```python
from build123d import *

# Parameters (mm, degrees)
SKETCH_1_W                                 = 300
SKETCH_1_H                                 = 120
EXTRUDE_1_DEPTH                            = 100
EXTRUDE_2_DEPTH                            = 20
FILLET_2_R                                 = 10
FILLET_3_R                                 = 10
MIRROR_6_AT_THE_SECOND_PLANE_COPY_1_DEPTH  = 20
FILLET_10_R                                = 10
FILLET_11_R                                = 10
FILLET_12_R                                = 10
FILLET_13_R                                = 10
FILLET_14_R                                = 10
FILLET_15_R                                = 10
CUT_EXTRUDE_1_REACH                        = 258.744
PATTERN_LINEAR_1_COUNT                     = 4
PATTERN_LINEAR_1_PITCH                     = 40
PATTERN_LINEAR_1_COL_COUNT                 = 4
PATTERN_LINEAR_1_COL_PITCH                 = 40
SKETCH_4_R                                 = 30
EXTRUDE_3_DEPTH                            = 13
SKETCH_6_R                                 = 32.5
CUT_EXTRUDE_2_DEPTH                        = 283.853914089
FILLET_16_R                                = 5
CUT_EXTRUDE_6_DEPTH                        = 399.453619326
CUT_EXTRUDE_6_DEPTH_BACK                   = 10
SKETCH_10_W                                = 239.935229407
SKETCH_10_H                                = 310.477115034
SKETCH_11_R                                = 2
CUT_EXTRUDE_7_DEPTH                        = 10
MIRROR_8_AT_THE_SECOND_PLANE_COPY_1_SKET_R = 2
MIRROR_8_AT_THE_SECOND_PLANE_COPY_1_DEPTH  = 10
SKETCH_12_R                                = 2
CUT_EXTRUDE_8_DEPTH                        = 261.089093804
PATTERN_CIRCULAR_2_COUNT                   = 6


with BuildPart() as part:
    # 草图1 → 凸台-拉伸1 (new body)
    with BuildSketch(Plane.XY):
        Rectangle(SKETCH_1_W, SKETCH_1_H)
    extrude(amount=EXTRUDE_1_DEPTH)

    # 草图2 → 凸台-拉伸2 (add)
    with BuildSketch(Plane(origin=(0, 60, 0), x_dir=(1, 0, 0), z_dir=(0, 1, 0))):
        with BuildLine():
            Line((150, -50), (150, -40))
            ThreePointArc((150, -40), (228.729833462, -50), (150, -60))
            Line((150, -60), (150, -50))
        make_face()
    extrude_2 = extrude(amount=-EXTRUDE_2_DEPTH)

    # 圆角2
    fillet_2_edges = [part.edges().sort_by_distance(p)[0] for p in [
        (150, 50, 40),
    ]]
    fillet(fillet_2_edges, radius=FILLET_2_R)

    # 圆角3
    fillet_3_edges = [part.edges().sort_by_distance(p)[0] for p in [
        (150, 50, 60),
    ]]
    fillet(fillet_3_edges, radius=FILLET_3_R)

    # 镜向6: 凸台-拉伸2 across plane
    add(extrude_2.mirror(Plane(origin=(0, 0, 0), x_dir=(0, 0, 1), z_dir=(1, 0, 0))))

    # 镜向6 at the second plane: 凸台-拉伸2 across plane
    add(extrude_2.mirror(Plane.ZX))

    # 镜向6 at the second plane copy 1 sket → 镜向6 at the second plane copy 1 (add)
    with BuildSketch(Plane(origin=(0, -60, 0), x_dir=(-1, 0, 0), z_dir=(0, -1, 0))):
        with BuildLine():
            Line((150, -50), (150, -40))
            ThreePointArc((150, -40), (228.729833462, -50), (150, -60))
            Line((150, -60), (150, -50))
        make_face()
    extrude(amount=-MIRROR_6_AT_THE_SECOND_PLANE_COPY_1_DEPTH)

    # 圆角10
    fillet_10_edges = [part.edges().sort_by_distance(p)[0] for p in [
        (150, -50, 60),
    ]]
    fillet(fillet_10_edges, radius=FILLET_10_R)

    # 圆角11
    fillet_11_edges = [part.edges().sort_by_distance(p)[0] for p in [
        (150, -50, 40),
    ]]
    fillet(fillet_11_edges, radius=FILLET_11_R)

    # 圆角12
    fillet_12_edges = [part.edges().sort_by_distance(p)[0] for p in [
        (-150, 50, 40),
    ]]
    fillet(fillet_12_edges, radius=FILLET_12_R)

    # 圆角13
    fillet_13_edges = [part.edges().sort_by_distance(p)[0] for p in [
        (-150, -50, 60),
    ]]
    fillet(fillet_13_edges, radius=FILLET_13_R)

    # 圆角14
    fillet_14_edges = [part.edges().sort_by_distance(p)[0] for p in [
        (-150, 50, 60),
    ]]
    fillet(fillet_14_edges, radius=FILLET_14_R)

    # 圆角15
    fillet_15_edges = [part.edges().sort_by_distance(p)[0] for p in [
        (-150, -50, 40),
    ]]
    fillet(fillet_15_edges, radius=FILLET_15_R)

    # 草图3 → 切除-拉伸1 (cut, up to next)
    with BuildSketch(Plane.XY.offset(100), mode=Mode.PRIVATE) as cut_extrude_1_sk1:
        with BuildLine():
            Line((-11.916195323, -32.511613), (-11.916195323, 32.511613))
            ThreePointArc((-11.916195323, 32.511613), (0, 44.427808323), (11.916195323, 32.511613))
            Line((11.916195323, 32.511613), (11.916195323, -32.511613))
            ThreePointArc((11.916195323, -32.511613), (0, -44.427808323), (-11.916195323, -32.511613))
        make_face()
    cut_extrude_1_tool1 = extrude(cut_extrude_1_sk1.sketch, amount=-CUT_EXTRUDE_1_REACH, mode=Mode.PRIVATE) & part.part
    cut_extrude_1 = cut_extrude_1_tool1.solids().sort_by_distance((0, 0, 100))[0]
    add(cut_extrude_1, mode=Mode.SUBTRACT)

    # 阵列(线性)1: 切除-拉伸1 ×4
    with Locations(*[(i * PATTERN_LINEAR_1_PITCH, 0, 0) for i in range(1, PATTERN_LINEAR_1_COUNT)]):
        add(cut_extrude_1, mode=Mode.SUBTRACT)

    # 阵列(线性)1 col: 切除-拉伸1 ×4
    with Locations(*[(-i * PATTERN_LINEAR_1_COL_PITCH, 0, 0) for i in range(1, PATTERN_LINEAR_1_COL_COUNT)]):
        add(cut_extrude_1, mode=Mode.SUBTRACT)

    # 草图4 → 凸台-拉伸3 (add)
    with BuildSketch(Plane.XZ.offset(60)):
        with Locations(Location((188.729833462, 50, 0), (0, 0, 90))):
            Circle(SKETCH_4_R)
    extrude(amount=EXTRUDE_3_DEPTH)

    # 草图6 → 切除-拉伸2 (cut, through all)
    with BuildSketch(Plane(origin=(0, 60, 0), x_dir=(1, 0, 0), z_dir=(0, 1, 0))):
        with Locations(Location((-188.729833462, -50, 0), (0, 0, 270))):
            Circle(SKETCH_6_R)
    extrude(amount=-CUT_EXTRUDE_2_DEPTH, mode=Mode.SUBTRACT)

    # 圆角16
    fillet_16_edges = [part.edges().sort_by_distance(p)[0] for p in [
        (-150, 0, 100),
        (0, -60, 100),
        (150, 0, 100),
        (0, -60, 0),
        (-150, 0, 0),
        (0, 60, 0),
        (150, 0, 0),
        (0, 60, 100),
    ]]
    fillet(fillet_16_edges, radius=FILLET_16_R)

    # 草图10 → 切除-拉伸6 (cut, two sides: drawn at the far end of the back side and taken through both)
    with BuildSketch(Plane.ZY.offset(150).offset(-CUT_EXTRUDE_6_DEPTH_BACK)):
        with Locations((-5.422984107, 66.466365428)):
            Rectangle(SKETCH_10_W, SKETCH_10_H)
    extrude(amount=CUT_EXTRUDE_6_DEPTH + CUT_EXTRUDE_6_DEPTH_BACK, mode=Mode.SUBTRACT)

    # 草图11 → 切除-拉伸7 (cut)
    with BuildSketch(Plane.ZY.offset(140)):
        with Locations(Location((90, 55.461, 0), (0, 0, 270))):
            Circle(SKETCH_11_R)
    cut_extrude_7 = extrude(amount=-CUT_EXTRUDE_7_DEPTH, mode=Mode.SUBTRACT)

    # 镜向8: 切除-拉伸7 across plane
    add(cut_extrude_7.mirror(Plane.ZX), mode=Mode.SUBTRACT)

    # 镜向8 at the second plane: 切除-拉伸7 across plane
    add(cut_extrude_7.mirror(Plane.XY.offset(50)), mode=Mode.SUBTRACT)

    # 镜向8 at the second plane copy 1 sket → 镜向8 at the second plane copy 1 (cut)
    with BuildSketch(Plane(origin=(-140, 0, 100), x_dir=(0, 0, -1), z_dir=(-1, 0, 0))):
        with Locations(Location((90, 55.461, 0), (0, 0, 270))):
            Circle(MIRROR_8_AT_THE_SECOND_PLANE_COPY_1_SKET_R)
    extrude(amount=-MIRROR_8_AT_THE_SECOND_PLANE_COPY_1_DEPTH, mode=Mode.SUBTRACT)

    # 草图12 → 切除-拉伸8 (cut, through all)
    with BuildSketch(Plane(origin=(0, 0, 0), x_dir=(1, 0, 0), z_dir=(0, 1, 0))):
        with Locations(Location((188.729833462, -32.75, 0), (0, 0, 90))):
            Circle(SKETCH_12_R)
    cut_extrude_8 = extrude(amount=CUT_EXTRUDE_8_DEPTH, mode=Mode.SUBTRACT)

    # 阵列(圆周)2: 切除-拉伸8 ×6 about axis
    pattern_circular_2_axis = Axis((188.729833462, 0, 50), (0, 1, 0))
    for i in range(1, PATTERN_CIRCULAR_2_COUNT):
        add(cut_extrude_8.rotate(pattern_circular_2_axis, i * 360 / PATTERN_CIRCULAR_2_COUNT), mode=Mode.SUBTRACT)


solid = part.part
```
Read the model definition and answer for the solid it produces. Units are mm, in the model's axes. A direction names the side the tool comes from. Coordinates: 2 decimals unless noted, no trailing zeros. Write each loop counter-clockwise with the first axis right and the second up, starting at its lowest first coordinate (ties: lowest second). Pieces come first, ordered by that corner, then holes. Notation, with made-up numbers: (83.5, 4) -> (132.5, 4) arc R16 cw to (132.5, 10) -> close; hole circle Ø2 at (56.5, -1.5). An arc over 180 degrees is marked (long way). Write item = value, one per line.
(1) Given pin 1 Ø6.5 at (y, z) = (55.461, 90) entering from +X; pin 2 Ø19.5 at (y, z) = (10.5, 67.5) entering from +X; pin 3 Ø1.5 at (x, z) = (38, 13) entering from -Y, each flat-ended and moving along its own axis, determine where each tip first touches the part or whether it passes through.
From the geometry:
pin_1 = 204.52
pin_2 = 150
pin_3 = -60
(2) Which of the six approach directions +Z, -Z, +X, -X, +Y, -Y give full straight-line access (tool end or side, diameter ignored) to faces 1 (the face through (39.738, 44.425, 50.7)), 2 (the face through (155.25, -49.86, 17.88))?
From the geometry:
face_1 = +Z, -Z
face_2 = -Z, +Y, -Y
(3) Section A-A on x = -80 is taken. Write down the section's boundary in (y, z), plus the area to 3 significant figures.
From the geometry:
outline = (-60, 5) arc R5 ccw to (-55, 0) -> (-44.43, 0) -> (-44.43, 100) -> (-55, 100) arc R5 ccw to (-60, 95) -> close; (44.43, 0) -> (55, 0) arc R5 ccw to (60, 5) -> (60, 95) arc R5 ccw to (55, 100) -> (44.43, 100) -> close
area = 3,090 mm2
(4) Section C-C on x = 97 is taken. Write down the section's boundary in (y, z), plus the area to 3 significant figures.
From the geometry:
outline = (-60, 5) arc R5 ccw to (-55, 0) -> (55, 0) arc R5 ccw to (60, 5) -> (60, 95) arc R5 ccw to (55, 100) -> (-55, 100) arc R5 ccw to (-60, 95) -> close
area = 12,000 mm2
(5) For a pull along X with two mould halves and no side action, classify faces 3 (the face through (168.454, -66.409, 27.889)), 4 (the face through (40.262, -44.425, 50.7)), 5 (the face through (155.25, 49.86, 17.88)), 6 (the face through (190, 40, 49)) as +X half, -X half, draft (parallel to the pull), parting line (faces both ways), or undercut.
From the geometry:
face_3 = parting line
face_4 = undercut
face_5 = undercut
face_6 = draft
(6) Section B-B on y = -48.5 is taken. Write down the section's boundary in (x, z), plus the area to 3 significant figures.
From the geometry:
outline = (-140, 0) -> (145, 0) arc R5 ccw to (150, 5) -> (150, 9.08) arc R10 cw to (165.75, 17.26) arc R40 ccw (long way) to (165.75, 82.74) arc R10 cw to (150, 90.92) -> (150, 95) arc R5 ccw to (145, 100) -> (-140, 100) -> close
area = 34,300 mm2
(7) Straight lines are drawn through the part: L1, parallel to Y at x = -132.5, z = 10; L2, parallel to Y at x = 39.5, z = 46; L3, parallel to Y at x = 192.5, z = 70.5. For each, find the intervals that lie inside material, in ascending order. Write a range as from..to.
From the geometry:
L1 = -60..-57.46, -53.46..53.46, 57.46..60
L2 = -60..-44.42, 44.42..60
L3 = -73..-40, 40..60
(8) Section D-D on z = 50 is taken. Count the separate pieces of the cut face and the enclosed holes in it, plus the area to 3 significant figures.
From the geometry:
separate_pieces = 1
enclosed_holes = 7
area = 24,800 mm2
